from build123d import *

# Parameters (mm, degrees)
SKETCH1_W           = 48
SKETCH1_H           = 18
BOSS_EXTRUDE1_DEPTH = 0.8
FILLET1_R           = 0.1
SKETCH3_W           = 7.7
SKETCH3_H           = 7.7
BOSS_EXTRUDE2_DEPTH = 2.5


with BuildPart() as part:
    # Sketch1 → Boss-Extrude1 (new, symmetric)
    with BuildSketch(Plane(origin=(0, 0, 0), x_dir=(1, 0, 0), z_dir=(0, 1, 0))):
        Rectangle(SKETCH1_W, SKETCH1_H)
    extrude(amount=BOSS_EXTRUDE1_DEPTH, both=True)

    # Fillet1
    fillet1_edges = [part.edges().sort_by_distance(p)[0] for p in [
        (24, 0, 9),
        (-24, 0, 9),
        (-24, 0, -9),
        (24, 0, -9),
    ]]
    fillet(fillet1_edges, radius=FILLET1_R)

    # Sketch3 → Boss-Extrude2 (add)
    with BuildSketch(Plane(origin=(0, 0.8, 0), x_dir=(1, 0, 0), z_dir=(0, 1, 0))):
        with Locations((-20.15, 0)):
            Rectangle(SKETCH3_W, SKETCH3_H)
    extrude(amount=BOSS_EXTRUDE2_DEPTH)


solid = part.part
Verification items for the finished model (mm, model axes). A direction names the side the tool comes from. Give positions to 0.01 mm unless a question says otherwise; leave off trailing zeros. Write each loop counter-clockwise with the first axis right and the second up, starting at its lowest first coordinate (ties: lowest second). Pieces come first, ordered by that corner, then holes. Notation, with made-up numbers: M 5,-32 L 34,-32 A31 cw 34,7 Z; hole C -35,40.5 d6. An arc over 180 degrees is marked long. Put each result on its own line as item: value. Start each with the question number.
1. Section check A-A (z = -0.75). Record the cut outline in (x, y).
2. Set-up check for faces 1 (the face through (-20, 2, -3.85)), 2 (the face through (-20, 2, 3.85)), 3 (the face through (-16.3, 2, 0)): record each of +Z, -Z, +X, -X, +Y, -Y from which the full face is reachable in a straight line by a thin tool's end or side.
3. Section check C-C (x = 4). Record the cut outline in (y, z), and give its area (3 significant figures).
4. Scan lines: line 1 along Y through (x, z) = (14, 1.5); line 2 along X through (y, z) = (2, -0.25). Record each from-to range of solid material in increasing order. Write a range as [from, to].
5. Go/stop test with flat-tipped pins: pin 1 Ø0.8 at (x, y) = (-20.5, 1.5) entering from -Z; pin 2 Ø2 at (x, z) = (-10.5, -2.5) entering from +Y; pin 3 Ø0.8 at (x, y) = (-19, 2) entering from +Z. Record where each tip stops, or that it passes through.
6. Section check B-B (y = 1.35). Record the cut outline in (x, z).
Answer list:
1. outline: M -24,-0.8 L 24,-0.8 L 24,0.8 L -16.3,0.8 L -16.3,3.3 L -24,3.3 Z
2. face 1: -Z, +X, -X, +Y
2. face 2: +Z, +X, -X, +Y
2. face 3: +Z, -Z, +X, +Y
3. outline: M -0.8,-9 L 0.8,-9 L 0.8,9 L -0.8,9 Z
3. area: 28.8 mm2
4. line 1: [-0.8, 0.8]
4. line 2: [-24, -16.3]
5. pin 1: z = -3.85
5. pin 2: y = 0.8
5. pin 3: z = 3.85
6. outline: M -24,-3.85 L -16.3,-3.85 L -16.3,3.85 L -24,3.85 Z
